Geometry: final body of the model. Coordinates: model frame, mm. A direction names the side the tool comes from. Coordinates: 2 decimals unless noted, no trailing zeros. Order: outer loops, then holes, each group sorted by start corner. A loop starts at its lowest first (then second) coordinate and runs counter-clockwise, first axis right, second up. Notation, with made-up numbers: (-34.75, 85.5) -> (21.25, 85.5) arc R34 ccw to (21.25, 119.5) -> close; hole circle Ø3 at (52.5, 72). An arc over 180 degrees is marked (long way). Use one line per item in the form item = value.
```python
from build123d import *

# Parameters (mm, degrees)
SKETCH1_W           = 26.67
SKETCH1_H           = 24.765
BOSS_EXTRUDE1_DEPTH = 102.87
FILLET1_R           = 5.08
SKETCH2_W           = 11.43
SKETCH2_H           = 4.445
CUT_EXTRUDE1_DEPTH  = 12.7


with BuildPart() as part:
    # Sketch1 → Boss-Extrude1 (new body)
    with BuildSketch(Plane.XY):
        Rectangle(SKETCH1_W, SKETCH1_H)
    extrude(amount=BOSS_EXTRUDE1_DEPTH)

    # Fillet1
    fillet1_edges = [part.edges().sort_by_distance(p)[0] for p in [
        (13.335, 0, 102.87),
        (0, 12.3825, 102.87),
        (-13.335, 0, 102.87),
        (0, 12.3825, 0),
        (13.335, 0, 0),
        (0, -12.3825, 0),
        (-13.335, 0, 0),
        (-13.335, 12.3825, 51.435),
        (13.335, 12.3825, 51.435),
        (13.335, -12.3825, 51.435),
        (-13.335, -12.3825, 51.435),
        (0, -12.3825, 102.87),
    ]]
    fillet(fillet1_edges, radius=FILLET1_R)

    # Sketch2 → Cut-Extrude1 (cut)
    with BuildSketch(Plane(origin=(0, 0, 0), x_dir=(-1, 0, 0), z_dir=(0, 0, -1))):
        with Locations((0, -2.54)):
            Rectangle(SKETCH2_W, SKETCH2_H)
        Polygon((-2.54, 2.2225), (2.54, 2.2225), (3.4925, 3.4925), (3.4925, 4.7625), (-3.4925, 4.7625), (-3.4925, 3.4925), align=None)
    extrude(amount=-CUT_EXTRUDE1_DEPTH, mode=Mode.SUBTRACT)


solid = part.part
```
1) Material intervals for probe 1 along X at (y, z) = (-2.5, 10) (3 decimals); probe 2 along Y at (x, z) = (8.5, 26); probe 3 along X at (y, z) = (-10.25, 29.5), sorted ascending. Write a range as from..to.
Results found:
probe_1 = -13.335..-5.715, 5.715..13.335
probe_2 = -12.38..12.38
probe_3 = -12.39..12.39
2) Pull-direction query (X, two-part tool) for faces 1 (the cylindrical face through (11.81, -10.93, 52.08)), 2 (the cylindrical face through (-11.89, -10.85, 52.08)), 3 (the flat face through (0, 0, 0)), 4 (the flat face through (0, -0.317, 6)); classes: released by +X, released by -X, zero draft, split by the parting line, or undercut.
Results found:
face_1 = released by +X
face_2 = released by -X
face_3 = zero draft
face_4 = undercut
3) Section C-C, the plane z = 23. Output: boundary loops of the cut face in (x, y) (1 decimal).
Results found:
outline = (-13.3, -7.3) arc R5.1 ccw to (-8.3, -12.4) -> (8.3, -12.4) arc R5.1 ccw to (13.3, -7.3) -> (13.3, 7.3) arc R5.1 ccw to (8.3, 12.4) -> (-8.3, 12.4) arc R5.1 ccw to (-13.3, 7.3) -> close
4) Section D-D, the plane x = 10.5. Output: boundary loops of the cut face in (y, z).
Results found:
outline = (-11.86, 5.08) arc R4.56 ccw to (-7.3, 0.52) -> (7.3, 0.52) arc R4.56 ccw to (11.86, 5.08) -> (11.86, 97.79) arc R4.56 ccw to (7.3, 102.35) -> (-7.3, 102.35) arc R4.56 ccw to (-11.86, 97.79) -> close
5) Contact query for flat-ended pins moving along their axis: P1, Ø2, axis at x = 1, y = 3.5, coming from the -Z side; P2, Ø2, axis at y = -3.5, z = 3, coming from the +X side. Output: stop coordinate, or through.
Results found:
P1 = 12.7
P2 = 13.22
6) Access query for faces 5 (the flat face through (-5.715, -3, 6)), 6 (the cylindrical face through (0.116, -10.934, 101.342)). Directions: +Z, -Z, +X, -X, +Y, -Y. A direction counts if a zero-diameter tool reaches every point of the face in a straight line with its end or side. Return the directions, or none.
Results found:
face_5 = -Z
face_6 = +Z, +X, -X, -Y
7) Section B-B, the plane x = 4.5. Output: boundary loops of the cut face in (y, z).
Results found:
outline = (-12.38, 5.08) arc R5.08 ccw to (-7.3, 0) -> (-4.76, 0) -> (-4.76, 12.7) -> (-0.32, 12.7) -> (-0.32, 0) -> (7.3, 0) arc R5.08 ccw to (12.38, 5.08) -> (12.38, 97.79) arc R5.08 ccw to (7.3, 102.87) -> (-7.3, 102.87) arc R5.08 ccw to (-12.38, 97.79) -> close
8) Section A-A, the plane z = 9.5. Output: boundary loops of the cut face in (x, y) (1 decimal).
Results found:
outline = (-13.3, -7.3) arc R5.1 ccw to (-8.3, -12.4) -> (8.3, -12.4) arc R5.1 ccw to (13.3, -7.3) -> (13.3, 7.3) arc R5.1 ccw to (8.3, 12.4) -> (-8.3, 12.4) arc R5.1 ccw to (-13.3, 7.3) -> close; hole (-5.7, -4.8) -> (5.7, -4.8) -> (5.7, -0.3) -> (-5.7, -0.3) -> close; hole (-3.5, 3.5) -> (-2.5, 2.2) -> (2.5, 2.2) -> (3.5, 3.5) -> (3.5, 4.8) -> (-3.5, 4.8) -> close
